Here's the drawing with two shaded views (mm, measured from the low corner). I have some questions. A direction names the side the tool comes from. Round coordinates to 2 decimals unless told otherwise and drop trailing zeros. Order: outer loops, then holes, each group sorted by start corner. A loop starts at its lowest first (then second) coordinate and runs counter-clockwise, first axis right, second up. Notation, with made-up numbers: (21.25, 44) - (60.25, 44) arc R10 cw to (60.25, 52) - close; hole circle Ø4 at (16.25, 59.25). An arc over 180 degrees is marked (long way). One line per item, written item: value.
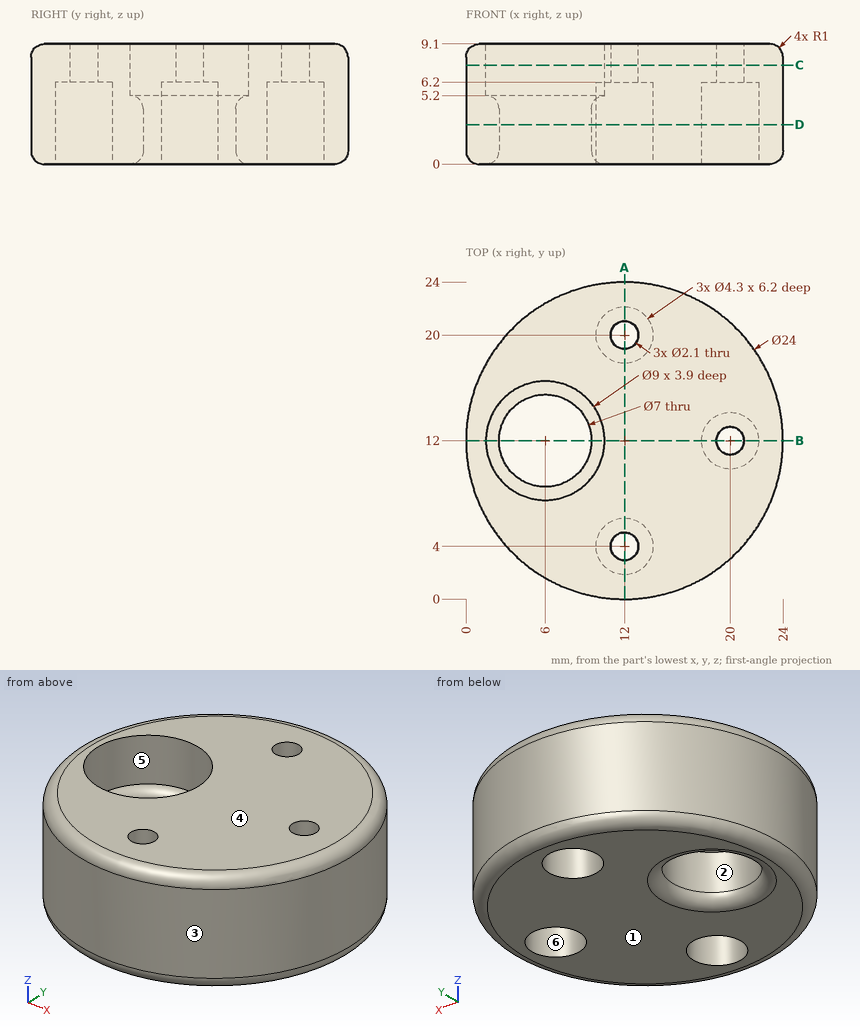
Q1. If I drill on line 1 along Y through (x, z) = (12, 4); line 2 along Y through (x, z) = (11.5, 8.5); line 3 along Y through (x, z) = (20.75, 1.75) (1 decimal), over which ranges is the centre line in solid material (lowest first)?
Results list:
line 1: 0 to 1.85, 6.15 to 17.85, 22.15 to 24
line 2: 0.09 to 3.08, 4.92 to 19.08, 20.92 to 23.91
line 3: 3.8 to 10, 14 to 20.2
Q2. Which directions (+Z, -Z, +X, -X, +Y, -Y) give clear straight access to the entire face, cutting with the end or side of a thin tool? Please do the marked faces 4, 5 and 6.
Results list:
face 4: +Z, +X, -X, +Y, -Y
face 5: +Z
face 6: -Z
Q3. Will these pins go through, and if not, where does the flat tip stop? pin 1 (2.5 mm diameter, centred on x = 12, y = 20, fed in from -Z); pin 2 (1.7 mm diameter, centred on x = 20, y = 12, fed in from -Z); pin 3 (1.5 mm diameter, centred on x = 16.5, z = 1, fed in from +Y).
Results list:
pin 1: z = 6.2
pin 2: through
pin 3: y = 23.4
Q4. If we section it at D-D, the plane z = 3: Please give me the cut outline in (x, y).
Results list:
outline: circle Ø24 at (12, 12); hole circle Ø7 at (6, 12); hole circle Ø4.3 at (12, 4); hole circle Ø4.3 at (12, 20); hole circle Ø4.3 at (20, 12)
Q5. If we section it at C-C, the plane z = 7.5: Please give me the cut outline in (x, y), then the cut area to 3 significant figures.
Results list:
outline: circle Ø24 at (12, 12); hole circle Ø9 at (6, 12); hole circle Ø2.1 at (12, 4); hole circle Ø2.1 at (12, 20); hole circle Ø2.1 at (20, 12)
area: 378 mm²
Q6. If we section it at B-B, the plane y = 12: Give the number of separate pieces and of enclosed holes in the cut face, then the cut area to 3 significant figures.
Results list:
separate pieces: 3
enclosed holes: 0
area: 112 mm²
Q7. If we section it at A-A, the plane x = 12: Please give me the cut outline in (y, z), then the cut area to 3 significant figures.
Results list:
outline: (0, 1) arc R1 ccw to (1, 0) - (1.85, 0) - (1.85, 6.2) - (2.95, 6.2) - (2.95, 9.1) - (1, 9.1) arc R1 ccw to (0, 8.1) - close; (5.05, 6.2) - (6.15, 6.2) - (6.15, 0) - (17.85, 0) - (17.85, 6.2) - (18.95, 6.2) - (18.95, 9.1) - (5.05, 9.1) - close; (21.05, 6.2) - (22.15, 6.2) - (22.15, 0) - (23, 0) arc R1 ccw to (24, 1) - (24, 8.1) arc R1 ccw to (23, 9.1) - (21.05, 9.1) - close
area: 152 mm²
Q8. We'd pull the mould along X, two halves only. Please class the marked faces 1, 2 and 3: released by +X, released by -X, zero draft, split by the parting line, or undercut.
Results list:
face 1: zero draft
face 2: undercut
face 3: split by the parting line
